Autodesk Fusion 360 part; units mm, degrees
sketch "Sketch1" plane through (0, 0, 0) normal (0, 1, 0) x (1, 0, 0)
  line L0 (0, 0) -> (33.5, 0)
  line L1 (33.5, 0) -> (33.5, -11.5)
  line L2 (33.5, -11.5) -> (0, -11.5)
  line L3 (0, -11.5) -> (0, 0)
  line L4 (12.8, -9) -> (20.7, -9)
  line L5 (20.7, -9) -> (20.7, -5.6)
  line L6 (20.7, -5.6) -> (12.8, -5.6)
  line L7 (12.8, -5.6) -> (12.8, -9)
  line L8 (12.3, -9.5) -> (21.2, -9.5)
  line L9 (21.2, -9.5) -> (21.2, -5.1)
  line L10 (21.2, -5.1) -> (12.3, -5.1)
  line L11 (12.3, -5.1) -> (12.3, -9.5)
  line L12 (3.5, -5.8) -> (6.5, -5.8)
  line L13 (6.5, -5.8) -> (6.5, -4.3)
  line L14 (6.5, -4.3) -> (3.5, -4.3)
  line L15 (3.5, -4.3) -> (3.5, -5.8)
  line L16 (27, -5.8) -> (30, -5.8)
  line L17 (30, -5.8) -> (30, -4.3)
  line L18 (30, -4.3) -> (27, -4.3)
  line L19 (27, -4.3) -> (27, -5.8)
  line L20 (2, -8.1) -> (7, -8.1)
  line L21 (7, -8.1) -> (7, -6.1)
  line L22 (7, -6.1) -> (2, -6.1)
  line L23 (2, -6.1) -> (2, -8.1)
  line L24 (2, -4) -> (7, -4)
  line L25 (7, -4) -> (7, -2)
  line L26 (7, -2) -> (2, -2)
  line L27 (2, -2) -> (2, -4)
  line L28 (26.5, -8.1) -> (31.5, -8.1)
  line L29 (31.5, -8.1) -> (31.5, -6.1)
  line L30 (31.5, -6.1) -> (26.5, -6.1)
  line L31 (26.5, -6.1) -> (26.5, -8.1)
  line L32 (26.5, -4) -> (31.5, -4)
  line L33 (31.5, -4) -> (31.5, -2)
  line L34 (31.5, -2) -> (26.5, -2)
  line L35 (26.5, -2) -> (26.5, -4)
  dimension "d1" = 7.9
  dimension "d2" = 3.4
  dimension "d3" = 8.9
  dimension "d4" = 4.4
  dimension "d5" = 0.5
  dimension "d6" = 0.5
  dimension "d7" = 3
  dimension "d8" = 1.5
  dimension "d9" = 3
  dimension "d10" = 1.5
  dimension "d12" = 0.2
  dimension "d14" = 0.2
  dimension "d15" = 5
  dimension "d16" = 2
  dimension "d17" = 0.3
  dimension "d18" = 1.5
  dimension "d19" = 5
  dimension "d20" = 2
  dimension "d21" = 1.5
  dimension "d22" = 0.3
  dimension "d23" = 5
  dimension "d24" = 2
  dimension "d25" = 5
  dimension "d26" = 2
  dimension "d27" = 0.5
  dimension "d28" = 0.3
  dimension "d29" = 0.3
  dimension "d30" = 0.5
  dimension "d31" = 2
  dimension "d32" = 2
  dimension "d33" = 2
  dimension "d34" = 2
  dimension "d49" = 20.5
  dimension "d50" = 6.3
extrude "Extrude1" add sketch "Sketch1" along normal blind 1 contours L0 L1 L2 L3 | L8 L9 L10 L11 | L12 L13 L14 L15 | L16 L17 L18 L19 | L20 L21 L22 L23 | L24 L25 L26 L27 | L28 L29 L30 L31 | L32 L33 L34 L35
extrude "Extrude2" add sketch "Sketch1" against normal blind 1 contours L8 L9 L10 L11
extrude "Extrude3" add sketch "Sketch1" against normal blind 5 contours L20 L21 L22 L23 | L24 L25 L26 L27 | L28 L29 L30 L31 | L32 L33 L34 L35
sketch "Sketch2" plane through (0, 0, 8.1) normal (0, 0, 1) x (-1, 0, 0)
  line L0 (-7, 0) -> (-2, 0)
  line L1 (-2, 0) -> (-2, 5)
  line L2 (-2, 5) -> (-7, 5)
  line L3 (-7, 5) -> (-7, 0)
  circle A0 centre (-5, 2.5) radius 1.6
  line L4 (-33.5, 0) -> (0, 0)
  circle A1 centre (-28.5, 2.5) radius 1.6
  line L5 (-31.5, 0) -> (-31.5, 5)
  line L6 (-26.5, 0) -> (-26.5, 5)
  dimension "d41" = 3.2
  dimension "d43" = 2.5
  dimension "d44" = 3.2
  dimension "d46" = 2.5
  dimension "d51" = 2
  dimension "d52" = 2
extrude "Extrude4" cut sketch "Sketch2" against normal blind 8 contours A0 | A1
equation "d50 = 5.8 mm + 0.5 mm"
Verification items for the finished model (mm, model axes). A direction names the side the tool comes from. Coordinates: 2 decimals unless noted, no trailing zeros. Order: outer loops, then holes, each group sorted by start corner. A loop starts at its lowest first (then second) coordinate and runs counter-clockwise, first axis right, second up. Notation, with made-up numbers: (14, 28.25) -> (48, 28.25) arc R20 ccw to (48, 66.25) -> close; hole circle Ø10 at (-15.75, 49). An arc over 180 degrees is marked (long way). Put each result on its own line as item: value. Start each with the question number.
1. Cross-section at B-B, the plane y = -2.5. Count the separate pieces of the cut face and the enclosed holes in it, then the cut area to 3 significant figures.
2. Go/stop test with flat-tipped pins: pin 1 Ø1.6 at (y, z) = (-3, 7.5) entering from +X; pin 2 Ø1.5 at (x, y) = (29, -3.5) entering from -Z; pin 3 Ø1 at (x, z) = (5, 9) entering from -Y. Record where each tip stops, or that it passes through.
3. Cross-section at A-A, the plane x = 17.5. Record the boundary of the cut face in (y, z).
4. Mould release check, pull along X, two halves, no side actions. Record for faces 5 (the flat face through (16.8, -0.5, 5.1)), 6 (the cylindrical face through (29.77, -1.53, 3.01)), 7 (the flat face through (2, -2, 7)): released by +X, released by -X, zero draft, split by the parting line, or undercut.
5. Cross-section at C-C, the plane y = -0.35. Record the boundary of the cut face in (x, z), then the cut area to 3 significant figures.
6. Access from +Z, -Z, +X, -X, +Y, -Y to the whole of each face (thin tool, end or side, straight path). Record for faces 1 (the flat face through (16.7, -0.5, 9.5)), 2 (the flat face through (30, -1, 8.1)), 3 (the flat face through (17, 0, 9)), 4 (the flat face through (7, -2, 3)).
7. Material ranges on L1, parallel to X at y = -0.4, z = 7; L2, parallel to X at y = -2.5, z = 7.15; L3, parallel to Z at x = 5.5, y = -4.35, recorded low to high. Write a range as [from, to].
8. Cross-section at D-D, the plane z = 3. Record the boundary of the cut face in (x, y), then the cut area to 3 significant figures.
Computed:
1. separate pieces: 8
1. enclosed holes: 0
1. area: 14.4 mm2
2. pin 1: x = 31.5
2. pin 2: z = 2
2. pin 3: y = 0
3. outline: (-1, 5.1) -> (0, 5.1) -> (0, 0) -> (1, 0) -> (1, 5.6) -> (-1, 5.6) -> close; (-1, 9) -> (1, 9) -> (1, 11.5) -> (0, 11.5) -> (0, 9.5) -> (-1, 9.5) -> close
4. face 5: zero draft
4. face 6: undercut
4. face 7: released by -X
5. outline: (2, 2) -> (7, 2) -> (7, 4) -> (2, 4) -> close; (2, 6.1) -> (7, 6.1) -> (7, 8.1) -> (2, 8.1) -> close; (12.3, 5.1) -> (21.2, 5.1) -> (21.2, 9.5) -> (12.3, 9.5) -> close; (26.5, 2) -> (31.5, 2) -> (31.5, 4) -> (26.5, 4) -> close; (26.5, 6.1) -> (31.5, 6.1) -> (31.5, 8.1) -> (26.5, 8.1) -> close; hole (12.8, 5.6) -> (20.7, 5.6) -> (20.7, 9) -> (12.8, 9) -> close
5. area: 52.3 mm2
6. face 1: +Z, +X, -X, -Y
6. face 2: +Z, +X, -Y
6. face 3: +Y, -Y
6. face 4: +Z, -Z, -Y
7. L1: [2, 7], [12.3, 12.8], [20.7, 21.2], [26.5, 31.5]
7. L2: [2, 3.4], [6.6, 7], [26.5, 26.9], [30.1, 31.5]
7. L3: [2, 4], [6.1, 8.1]
8. outline: (0, 0) -> (2, 0) -> (2, -5) -> (7, -5) -> (7, 0) -> (26.5, 0) -> (26.5, -5) -> (31.5, -5) -> (31.5, 0) -> (33.5, 0) -> (33.5, 1) -> (0, 1) -> close; hole circle Ø3.2 at (5, -2.5); hole circle Ø3.2 at (28.5, -2.5)
8. area: 67.4 mm2
